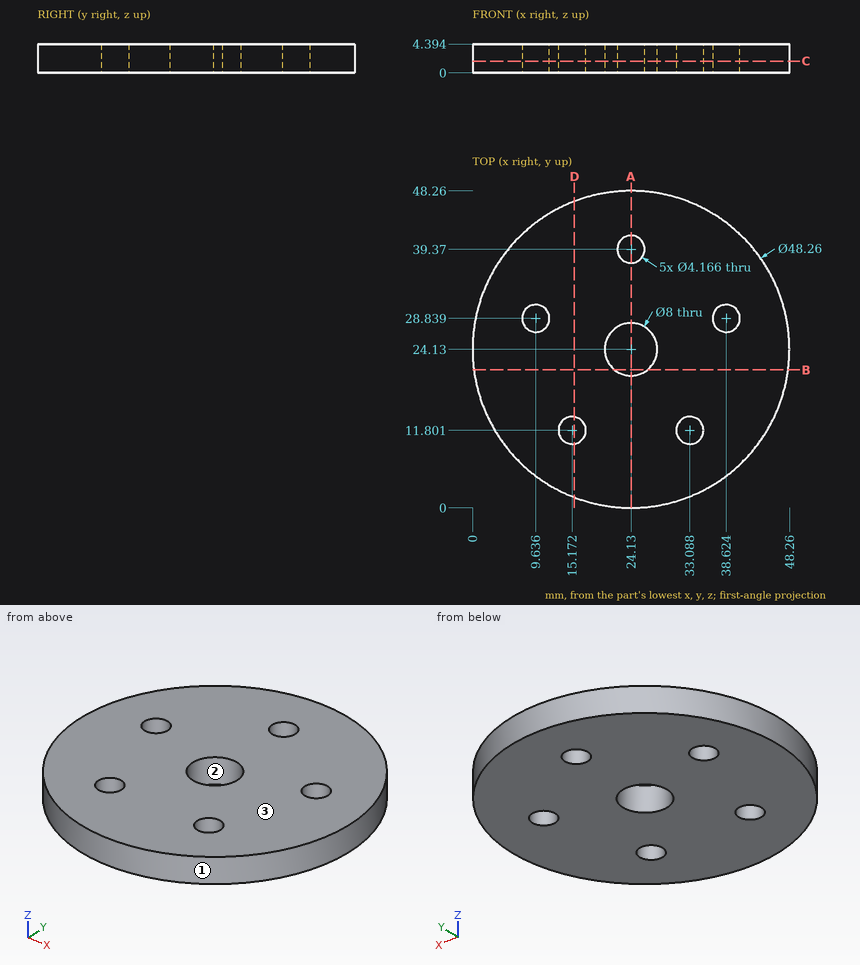
Can you work these out from the drawing? Everything is in mm from the part's minimum corner. Coordinates: 2 decimals unless noted, no trailing zeros. Loops run counter-clockwise (first coordinate to the right, second up) from the corner with the lowest first, then second, coordinate; pieces in that order, holes last.
1. Imagine slicing it at D-D, the plane x = 15.5. Please give me the cut outline in (y, z) (1 decimal), and give its area (3 significant figures).
2. If we mould it in two halves opening along Y, with no side actions, what happens to the marked faces 1, 2 and 3? For each: pulls with the +Y half, pulls with the -Y half, needs draft (parallel to the pull), parting line crosses it, or undercut.
3. Imagine slicing it at A-A, the plane x = 24.13. Please give me the cut outline in (y, z) (1 decimal).
4. Imagine slicing it at C-C, the plane z = 1.8. Please give me the cut outline in (x, y) (1 decimal).
5. I need wall thicknesses on L1, parallel to X at y = 24, z = 4; L2, parallel to X at y = 10, z = 0.9 (1 decimal); L3, parallel to Y at x = 9, z = 2.4 (1 decimal). Which ranges of each line are inside material? Lowest first, please.
6. For P1, Ø1, axis at x = 34, y = 27.5, coming from the -Z side; P2, Ø1, axis at x = 33.5, z = 1.5, coming from the -Y side, each with a flat end and sliding along its axis, tell me the tip position at first contact or that it passes through.
7. Imagine slicing it at B-B, the plane y = 21. Please give me the cut outline in (x, z) (1 decimal), and give its area (3 significant figures).
Taken from the geometry:
1. outline: (1.6, 0) - (9.7, 0) - (9.7, 4.4) - (1.6, 4.4) - close; (13.9, 0) - (46.7, 0) - (46.7, 4.4) - (13.9, 4.4) - close
1. area: 180 mm2
2. face 1: parting line crosses it
2. face 2: undercut
2. face 3: needs draft
3. outline: (0, 0) - (20.1, 0) - (20.1, 4.4) - (0, 4.4) - close; (28.1, 0) - (37.3, 0) - (37.3, 4.4) - (28.1, 4.4) - close; (41.5, 0) - (48.3, 0) - (48.3, 4.4) - (41.5, 4.4) - close
4. outline: circle Ø48.3 at (24.1, 24.1); hole circle Ø4.2 at (9.6, 28.8); hole circle Ø4.2 at (15.2, 11.8); hole circle Ø8 at (24.1, 24.1); hole circle Ø4.2 at (24.1, 39.4); hole circle Ø4.2 at (33.1, 11.8); hole circle Ø4.2 at (38.6, 28.8)
5. L1: x = 0 to 20.13, 28.13 to 48.26
5. L2: x = 4.6 to 14.1, 16.2 to 32, 34.1 to 43.7
5. L3: y = 5.3 to 26.9, 30.8 to 42.9
6. P1: stops at z = 0
6. P2: stops at y = 1.69
7. outline: (0.2, 0) - (21.6, 0) - (21.6, 4.4) - (0.2, 4.4) - close; (26.6, 0) - (48.1, 0) - (48.1, 4.4) - (26.6, 4.4) - close
7. area: 188 mm2
